from build123d import *
from OCP.BRepFilletAPI import BRepFilletAPI_MakeChamfer

# Parameters (mm, degrees)
SKETCH1_W            = 70
SKETCH1_H            = 17
SKETCH1_R            = 1
BOSS_EXTRUDE1_DEPTH  = 1.5
BOSS_EXTRUDE2_DEPTH  = 7.5
FILLET1_R            = 0.5
SKETCH3_R            = 1.75
CUT_EXTRUDE1_DEPTH   = 11
SKETCH4_W            = 4
SKETCH4_H            = 5.5
CUT_EXTRUDE2_DEPTH   = 7
FILLET1_OF_MIRROR1_R = 0.5
SKETCH5_W            = 19
SKETCH5_H            = 15
BOSS_EXTRUDE3_DEPTH  = 16.5
FILLET2_R            = 0.5
SKETCH6_W            = 6
SKETCH6_H            = 4.5
BOSS_EXTRUDE4_DEPTH  = 5
CHAMFER1_SIZE        = 2
CHAMFER1_SIZE2       = 0.535898385
SKETCH7_W            = 5
SKETCH7_H            = 2.5
BOSS_EXTRUDE5_DEPTH  = 8
CUT_EXTRUDE3_REACH   = 44.832
SKETCH8_W            = 0.5
SKETCH8_H            = 1


with BuildPart() as part:
    # Sketch1 → Boss-Extrude1 (new body)
    with BuildSketch(Plane(origin=(0, 0, 0), x_dir=(1, 0, 0), z_dir=(0, 1, 0))):
        Rectangle(SKETCH1_W, SKETCH1_H)
        with Locations(Location((-32.3, 6.2, 0), (0, 0, 270))):
            Circle(SKETCH1_R, mode=Mode.SUBTRACT)
        with Locations(Location((32.3, 6.2, 0), (0, 0, 270))):
            Circle(SKETCH1_R, mode=Mode.SUBTRACT)
        with Locations(Location((32.3, -6.2, 0), (0, 0, 270))):
            Circle(SKETCH1_R, mode=Mode.SUBTRACT)
        with Locations(Location((-32.3, -6.2, 0), (0, 0, 270))):
            Circle(SKETCH1_R, mode=Mode.SUBTRACT)
    extrude(amount=BOSS_EXTRUDE1_DEPTH)

    # Sketch2 → Boss-Extrude2 (add, symmetric)
    with BuildSketch(Plane.XY):
        Polygon((-31.2, 1.5), (-31.2, 9.5), (-30.350716041, 9.5), (-29.7, 15.5), (-23.7, 15.5), (-21.2, 6.5), (-21.2, 1.5), align=None)
    boss_extrude2 = extrude(amount=BOSS_EXTRUDE2_DEPTH, both=True)

    # Fillet1
    fillet1_edges = [part.edges().sort_by_distance(p)[0] for p in [
        (-31.2, 9.5, 0),
    ]]
    fillet(fillet1_edges, radius=FILLET1_R)

    # Sketch3 → Cut-Extrude1 (cut)
    with BuildSketch(Plane(origin=(0, 15.5, 0), x_dir=(1, 0, 0), z_dir=(0, 1, 0))):
        with Locations(Location((-26.7, 4.5, 0), (0, 0, 270))):
            Circle(SKETCH3_R)
        with Locations(Location((-26.7, 0, 0), (0, 0, 270))):
            Circle(SKETCH3_R)
        with Locations(Location((-26.7, -4.5, 0), (0, 0, 270))):
            Circle(SKETCH3_R)
    cut_extrude1 = extrude(amount=-CUT_EXTRUDE1_DEPTH, mode=Mode.SUBTRACT)

    # Sketch4 → Cut-Extrude2 (cut)
    with BuildSketch(Plane.ZY.offset(31.2)):
        with Locations((-4.5, 5.25)):
            Rectangle(SKETCH4_W, SKETCH4_H)
        with Locations((0, 5.25)):
            Rectangle(SKETCH4_W, SKETCH4_H)
        with Locations((4.5, 5.25)):
            Rectangle(SKETCH4_W, SKETCH4_H)
    cut_extrude2 = extrude(amount=-CUT_EXTRUDE2_DEPTH, mode=Mode.SUBTRACT)

    # Mirror1: Boss-Extrude2, Cut-Extrude1, Cut-Extrude2 across plane
    add(boss_extrude2.mirror(Plane(origin=(0, 0, 0), x_dir=(0, 0, 1), z_dir=(1, 0, 0))))
    add(cut_extrude1.mirror(Plane(origin=(0, 0, 0), x_dir=(0, 0, 1), z_dir=(1, 0, 0))), mode=Mode.SUBTRACT)
    add(cut_extrude2.mirror(Plane(origin=(0, 0, 0), x_dir=(0, 0, 1), z_dir=(1, 0, 0))), mode=Mode.SUBTRACT)

    # Fillet1 of Mirror1
    fillet1_of_mirror1_edges = [part.edges().sort_by_distance(p)[0] for p in [
        (31.2, 9.5, 0),
    ]]
    fillet(fillet1_of_mirror1_edges, radius=FILLET1_OF_MIRROR1_R)

    # Sketch5 → Boss-Extrude3 (add)
    with BuildSketch(Plane(origin=(0, 1.5, 0), x_dir=(1, 0, 0), z_dir=(0, 1, 0))):
        with Locations((10.7, 0)):
            Rectangle(SKETCH5_W, SKETCH5_H)
    extrude(amount=BOSS_EXTRUDE3_DEPTH)

    # Fillet2
    fillet2_edges = [part.edges().sort_by_distance(p)[0] for p in [
        (20.2, 9.75, 7.5),
        (20.2, 9.75, -7.5),
        (1.2, 9.75, -7.5),
        (1.2, 9.75, 7.5),
        (20.2, 18, 0),
        (10.7, 18, -7.5),
        (1.2, 18, 0),
        (10.7, 18, 7.5),
    ]]
    fillet(fillet2_edges, radius=FILLET2_R)

    # Sketch6 → Boss-Extrude4 (add)
    with BuildSketch(Plane(origin=(0, 1.5, 0), x_dir=(1, 0, 0), z_dir=(0, 1, 0))):
        with Locations((-13.2, 1.25)):
            Rectangle(SKETCH6_W, SKETCH6_H)
    extrude(amount=BOSS_EXTRUDE4_DEPTH)

    # Chamfer1: one chamfer whose edges measure the first distance from different faces: ONE call of the kernel's chamfer builder (chamfer() names one face for all edges)
    chamfer1_edges_1 = [part.edges().sort_by_distance(p)[0] for p in [
        (-16.2, 6.5, -1.25),
    ]]
    chamfer1_side_1 = [part.faces().sort_by_distance(p)[0] for p in [
        (-16.2, 4, -1.25),
    ]]
    chamfer1_edges_2 = [part.edges().sort_by_distance(p)[0] for p in [
        (-13.2, 6.5, 1),
    ]]
    chamfer1_side_2 = [part.faces().sort_by_distance(p)[0] for p in [
        (-13.2, 4, 1),
    ]]
    chamfer1_edges_3 = [part.edges().sort_by_distance(p)[0] for p in [
        (-10.2, 6.5, -1.25),
    ]]
    chamfer1_side_3 = [part.faces().sort_by_distance(p)[0] for p in [
        (-10.2, 4, -1.25),
    ]]
    chamfer1_edges_4 = [part.edges().sort_by_distance(p)[0] for p in [
        (-13.2, 6.5, -3.5),
    ]]
    chamfer1_side_4 = [part.faces().sort_by_distance(p)[0] for p in [
        (-13.2, 4, -3.5),
    ]]
    chamfer1 = BRepFilletAPI_MakeChamfer(part.part.solid().wrapped)
    for e in chamfer1_edges_1:
        chamfer1.Add(CHAMFER1_SIZE, CHAMFER1_SIZE2, e.wrapped, chamfer1_side_1[0].wrapped)  # the first distance lies on this face
    for e in chamfer1_edges_2:
        chamfer1.Add(CHAMFER1_SIZE, CHAMFER1_SIZE2, e.wrapped, chamfer1_side_2[0].wrapped)  # the first distance lies on this face
    for e in chamfer1_edges_3:
        chamfer1.Add(CHAMFER1_SIZE, CHAMFER1_SIZE2, e.wrapped, chamfer1_side_3[0].wrapped)  # the first distance lies on this face
    for e in chamfer1_edges_4:
        chamfer1.Add(CHAMFER1_SIZE, CHAMFER1_SIZE2, e.wrapped, chamfer1_side_4[0].wrapped)  # the first distance lies on this face
    add(Compound.cast(chamfer1.Shape()), mode=Mode.REPLACE)

    # Sketch7 → Boss-Extrude5 (add)
    with BuildSketch(Plane(origin=(0, 1.5, 0), x_dir=(1, 0, 0), z_dir=(0, 1, 0))):
        with Locations((-11.7, -7.15)):
            Rectangle(SKETCH7_W, SKETCH7_H)
    boss_extrude5 = extrude(amount=BOSS_EXTRUDE5_DEPTH)

    # Sketch8 → Cut-Extrude3 (cut, up to next)
    with BuildSketch(Plane.XY.offset(8.4), mode=Mode.PRIVATE) as cut_extrude3_sk1:
        with Locations((-13.95, 8.5)):
            Rectangle(SKETCH8_W, SKETCH8_H)
    cut_extrude3_tool1 = extrude(cut_extrude3_sk1.sketch, amount=-CUT_EXTRUDE3_REACH, mode=Mode.PRIVATE) & part.part
    # Sketch8 → Cut-Extrude3 (cut, up to next)
    with BuildSketch(Plane.XY.offset(8.4), mode=Mode.PRIVATE) as cut_extrude3_sk2:
        with BuildLine():
            Line((-12.2, 7.5), (-12.2, 9.5))
            Line((-12.2, 9.5), (-11.2, 9.5))
            Line((-11.2, 9.5), (-11.2, 7.5))
            ThreePointArc((-11.2, 7.5), (-11.7, 7), (-12.2, 7.5))
        make_face()
    cut_extrude3_tool2 = extrude(cut_extrude3_sk2.sketch, amount=-CUT_EXTRUDE3_REACH, mode=Mode.PRIVATE) & part.part
    # Sketch8 → Cut-Extrude3 (cut, up to next)
    with BuildSketch(Plane.XY.offset(8.4), mode=Mode.PRIVATE) as cut_extrude3_sk3:
        with Locations((-9.45, 8.5)):
            Rectangle(SKETCH8_W, SKETCH8_H)
    cut_extrude3_tool3 = extrude(cut_extrude3_sk3.sketch, amount=-CUT_EXTRUDE3_REACH, mode=Mode.PRIVATE) & part.part
    cut_extrude3_1 = cut_extrude3_tool1.solids().sort_by_distance((-13.95, 8.5, 8.4))[0]
    add(cut_extrude3_1, mode=Mode.SUBTRACT)
    cut_extrude3_2 = cut_extrude3_tool2.solids().sort_by_distance((-11.7, 8.301048, 8.4))[0]
    add(cut_extrude3_2, mode=Mode.SUBTRACT)
    cut_extrude3_3 = cut_extrude3_tool3.solids().sort_by_distance((-9.45, 8.5, 8.4))[0]
    add(cut_extrude3_3, mode=Mode.SUBTRACT)
    cut_extrude3 = cut_extrude3_1 + cut_extrude3_2 + cut_extrude3_3  # Cut-Extrude3 as one shape, for the pattern or mirror that repeats it

    # Mirror2: Boss-Extrude5, Cut-Extrude3 across plane
    add(boss_extrude5.mirror(Plane.XY))
    add(cut_extrude3.mirror(Plane.XY), mode=Mode.SUBTRACT)


solid = part.part
Model file for the job. Use its own axes, mm. A direction names the side the tool comes from. Give positions to 0.01 mm unless a question says otherwise; leave off trailing zeros. Order: outer loops, then holes, each group sorted by start corner. A loop starts at its lowest first (then second) coordinate and runs counter-clockwise, first axis right, second up. Notation, with made-up numbers: (-34, 29) -> (-18, 29) arc R23 ccw to (-18, 51) -> close; hole circle Ø1 at (50.25, 76). An arc over 180 degrees is marked (long way). Use CSV: the item, a comma, the result in double quotes.
1. Band-saw the part on B-B, the plane z = 4.5. Count the separate pieces of the cut face and the enclosed holes in it, then the cut area to 3 significant figures.
Outcome:
separate pieces,"3"
enclosed holes,"0"
area,"532 mm²"
2. Band-saw the part on D-D, the plane x = 0. Give the cut face in (y, z), then the cut area to 3 significant figures.
Outcome:
outline,"(0, -8.5) -> (1.5, -8.5) -> (1.5, 8.5) -> (0, 8.5) -> close"
area,"25.5 mm²"
3. Drop flat-ended pins along their axis: pin 1 (1.6 mm diameter, centred on x = -13.5, z = 7.5, fed in from +Y); pin 2 (3 mm diameter, centred on x = -29, y = 5, fed in from -Z); pin 3 (1.2 mm diameter, centred on y = 5, z = 0.5, fed in from +X); pin 4 (2 mm diameter, centred on x = -29, z = -4.5, fed in from -Y). Give the stop position or say it passes through.
Outcome:
pin 1,"y = 9.5"
pin 2,"z = -7.5"
pin 3,"x = 24.2"
pin 4,"y = 0"
4. 3-axis set-ups, long thin cutter, end or side, ignore diameter. For faces 1 (the flat face through (-10, 9.5, -7)), 2 (the flat face through (28, 5, 6.5)), 3 (the flat face through (-28, 5, -6.5)), 4 (the flat face through (-10.2, 3, -1)): which of +Z, -Z, +X, -X, +Y, -Y reach the whole face in a straight line?
Outcome:
face 1,"+Z, -Z, +Y"
face 2,"+X"
face 3,"-X"
face 4,"+Y"
5. Mould opens along X. For faces 5 (the flat face through (-24.2, 5, 0)), 6 (the flat face through (-29, 8, 4)), 7 (the flat face through (-13, 3, -3.5)) say: +X half, -X half, draft (parallel to the pull), parting line (faces both ways), or undercut.
Outcome:
face 5,"-X half"
face 6,"draft"
face 7,"undercut"
6. Drill centre lines: line 1 along Z through (x, y) = (26.7, 12.5); line 2 along X through (y, z) = (3.5, 0); line 3 along X through (y, z) = (6.25, -4). Where is each one in solid material? Low to high. Write a range as from..to.
Outcome:
line 1,"-7.5..-6.25, -2.75..-1.75, 1.75..2.75, 6.25..7.5"
line 2,"-24.2..-21.2, -16.2..-10.2, 1.2..20.2, 21.2..24.2"
line 3,"-24.2..-21.2, 1.2..20.2, 21.2..24.2"
7. Band-saw the part on C-C, the plane x = 9. Give the cut face in (y, z).
Outcome:
outline,"(0, -8.5) -> (1.5, -8.5) -> (1.5, -7.5) -> (17.5, -7.5) arc R0.5 ccw to (18, -7) -> (18, 7) arc R0.5 ccw to (17.5, 7.5) -> (1.5, 7.5) -> (1.5, 8.5) -> (0, 8.5) -> close"
